Autodesk Inventor part; units mm, degrees
ref_plane "YZ Plane" through (0, 0, 0) normal (1, 0, 0) x (0, 1, 0)
ref_plane "XZ Plane" through (0, 0, 0) normal (0, 1, 0) x (-1, 0, 0)
ref_plane "XY Plane" through (0, 0, 0) normal (0, 0, 1) x (1, 0, 0)
sketch "Sketch1" plane through (0, 0, 0) normal (0, 0, 1) x (1, 0, 0)
  line L0 (0, 0) -> (-40, 0)
  line L1 (-40, 0) -> (-40, 40)
  line L2 (-40, 40) -> (0, 40)
  line L3 (0, 40) -> (0, 0)
  line L4 (-30, 30) -> (-10, 30) construction
  line L5 (-10, 30) -> (-10, 10) construction
  line L6 (-10, 10) -> (-30, 10) construction
  line L7 (-30, 10) -> (-30, 30) construction
  line L8 (-30, 30) -> (-40, 30) construction
  line L9 (-10, 10) -> (0, 10) construction
  circle A0 centre (-30, 30) radius 2.6
  circle A1 centre (-10, 30) radius 2.6
  circle A2 centre (-10, 10) radius 2.6
  circle A3 centre (-30, 10) radius 2.6
  line L10 (-40, 40) -> (13, 40)
  line L11 (13, 40) -> (13, 100)
  line L12 (13, 100) -> (-40, 100)
  line L13 (-40, 100) -> (-40, 40)
  line L14 (13, 40) -> (0, 27)
  line L15 (-40, 100) -> (13, 100)
  line L16 (13, 100) -> (13, 120)
  line L17 (-40, 120) -> (-40, 100)
  line L18 (6.75, 120) -> (6.75, 112.72)
  line L19 (6.75, 112.72) -> (-33.75, 112.72)
  line L20 (-33.75, 112.72) -> (-33.75, 120)
  line L21 (-33.75, 112.72) -> (-40, 112.72) construction
  line L22 (6.75, 112.72) -> (13, 112.72) construction
  line L23 (-40, 120) -> (-33.75, 120)
  line L24 (13, 120) -> (6.75, 120)
  line L25 (-13.5, 112.72) -> (-13.5, 111.22) construction
  arc A4 (-18.2697, 112.72) -> (-8.7303, 112.72) centre (-13.5, 111.22) ccw
  dimension "d0" = 40
  dimension "d1" = 40
  dimension "d2" = 5.2
  dimension "d3" = 5.2
  dimension "d4" = 5.2
  dimension "d5" = 5.2
  dimension "d6" = 20
  dimension "d7" = 20
  dimension "d8" = 10
  dimension "d9" = 60
  dimension "d10" = 53
  dimension "d11" = 45
  dimension "d12" = 20
  dimension "d13" = 40.5
  dimension "d14" = 7.28
  dimension "d15" = 1.5
  dimension "d16" = 10
  dimension "d17" = 20
extrude "Extrusion1" add sketch "Sketch1" along normal blind 3.175 contours L0 L1 L2 L3 | L3 L10 L14 | L13 L12 L11 L10 L2 | L17 L23 L20 L19 A4 L18 L24 L16 L12
fillet "Fillet1" radius 3.175 4 edges at (0, 0, 1.5875) (-40, 0, 1.5875) (0, 27, 1.5875) (13, 40, 1.5875)
fillet "Fillet2" radius 0.5 4 edges at (13, 120, 1.5875) (-40, 120, 1.5875) (-33.75, 120, 1.5875) (6.75, 120, 1.5875)
sketch "Sketch2" plane through (0, 0, 3.175) normal (0, 0, 1) x (1, 0, 0)
  line L0 (13, 41.3151) -> (13, 119.5) construction
  line L1 (-40, 121.004) -> (13, 121.004) construction
  line L2 (13, 121.004) -> (13, 101.004) construction
  line L3 (13, 101.004) -> (-40, 101.004) construction
  line L4 (-40, 101.004) -> (-40, 121.004) construction
  circle A0 centre (-33.75, 106.36) radius 2.6
  circle A1 centre (6.75, 106.36) radius 2.6
  line L5 (-18.2697, 112.72) -> (-33.75, 112.72) construction
  line L6 (-33.75, 106.36) -> (-33.75, 112.72) construction
  line L7 (6.75, 112.72) -> (-8.7303, 112.72) construction
  line L8 (6.75, 106.36) -> (6.75, 112.72) construction
  point P0 (0, 0)
  dimension "d22" = 20
  dimension "d23" = 5.2
  dimension "d24" = 5.2
  dimension "d25" = 6.36
  dimension "d26" = 6.36
extrude "Extrusion2" cut sketch "Sketch2" against normal up to next
equation "\"d3\" = d2"
equation "\"d4\" = d2"
equation "\"d5\" = d2"
equation "\"d24\" = d23"
equation "\"d26\" = d25"
properties part number "X Axis Statonary Composite Belt Holder RIGHT"
Could you check a few things on this model? Use its own coordinates, in mm. A direction names the side the tool comes from. Round coordinates to 2 decimals unless told otherwise and drop trailing zeros. Write each loop counter-clockwise with the first axis right and the second up, starting at its lowest first coordinate (ties: lowest second). Pieces come first, ordered by that corner, then holes. Notation, with made-up numbers: M 54,13.5 L 67,13.5 A15 cw 67,42.5 Z; hole C 23,-36 d7. An arc over 180 degrees is marked long. Answer in a Markdown table with one row per item. Add a question column.
Q1. Imagine slicing it at D-D (z = 2.15). Please give me the cut outline in (x, y) (3 decimals).
Q2. If I drill on line 1 (X direction, y = 111.22, z = 2.3); line 2 (Y direction, x = -10, z = 1.1); line 3 (Y direction, x = -20.5, z = 1.4), over which ranges is the centre line in solid material (lowest first)? Write a range as from..to.
Q3. Imagine slicing it at B-B (x = -30). Please give me the cut outline in (y, z) (3 decimals).
Q4. Will these pins go through, and if not, where does the flat tip stop? pin 1 Ø4.5 at (x, y) = (-33.75, 106.36) entering from -Z; pin 2 Ø1 at (x, z) = (-1.5, 2) entering from +Y; pin 3 Ø1 at (y, z) = (12, 2) entering from +X.
Q5. On a 3-axis mill with a long thin cutter (end or side, diameter ignored), from which of +Z, -Z, +X, -X, +Y, -Y can I reach the whole of each face in a straight line? I mean faces 1 (the flat face through (-33.75, 116, 2)), 2 (the flat face through (0, 15, 2)), 3 (the flat face through (10, 120, 2)). Say none if no direction works.
Q6. Imagine slicing it at C-C (y = 111.22). Please give me the cut outline in (x, z) (3 decimals), then the cut area to 3 significant figures.
Q7. If we mould it in two halves opening along Y, with no side actions, what happens to faces 4 (the flat face through (-1, 112.72, 2)), 5 (the cylindrical face through (-8.8, 12.307, 1.565)), 6 (the flat face through (-20, 0, 2)), 7 (the flat face through (6.75, 116, 2))? For each: +Y half, -Y half, draft (parallel to the pull), parting line (faces both ways), or undercut.
Q8. Imagine slicing it at A-A (y = 10). Please give me the cut outline in (x, z) (3 decimals).
Values:
| question | item | result |
|---|---|---|
| 1 | outline | M -40,3.175 A3.175 ccw -36.825,0 L -3.175,0 A3.175 ccw 0,3.175 L 0,25.685 A3.175 cw 0.93,27.93 L 12.07,39.07 A3.175 ccw 13,41.315 L 13,119.5 A0.5 ccw 12.5,120 L 7.25,120 A0.5 ccw 6.75,119.5 L 6.75,112.72 L -8.73,112.72 A5 cw long -18.27,112.72 L -33.75,112.72 L -33.75,119.5 A0.5 ccw -34.25,120 L -39.5,120 A0.5 ccw -40,119.5 Z; hole C -33.75,106.36 d5.2; hole C -30,10 d5.2; hole C -30,30 d5.2; hole C -10,10 d5.2; hole C -10,30 d5.2; hole C 6.75,106.36 d5.2 |
| 2 | line 1 | -40..-18.5, -8.5..13 |
| 2 | line 2 | 0..7.4, 12.6..27.4, 32.6..107.65 |
| 2 | line 3 | 0..112.72 |
| 3 | outline | M 0,0 L 7.4,0 L 7.4,3.175 L 0,3.175 Z; M 12.6,0 L 27.4,0 L 27.4,3.175 L 12.6,3.175 Z; M 32.6,0 L 112.72,0 L 112.72,3.175 L 32.6,3.175 Z |
| 4 | pin 1 | through |
| 4 | pin 2 | y = 112.72 |
| 4 | pin 3 | x = 0 |
| 5 | face 1 | +Z, -Z, +Y |
| 5 | face 2 | +Z, -Z, +X, -Y |
| 5 | face 3 | +Z, -Z, +X, -X, +Y |
| 6 | outline | M -40,0 L -18.5,0 L -18.5,3.175 L -40,3.175 Z; M -8.5,0 L 13,0 L 13,3.175 L -8.5,3.175 Z |
| 6 | area | 137 mm^2 |
| 7 | face 4 | +Y half |
| 7 | face 5 | undercut |
| 7 | face 6 | -Y half |
| 7 | face 7 | draft |
| 8 | outline | M -40,0 L -32.6,0 L -32.6,3.175 L -40,3.175 Z; M -27.4,0 L -12.6,0 L -12.6,3.175 L -27.4,3.175 Z; M -7.4,0 L 0,0 L 0,3.175 L -7.4,3.175 Z |
